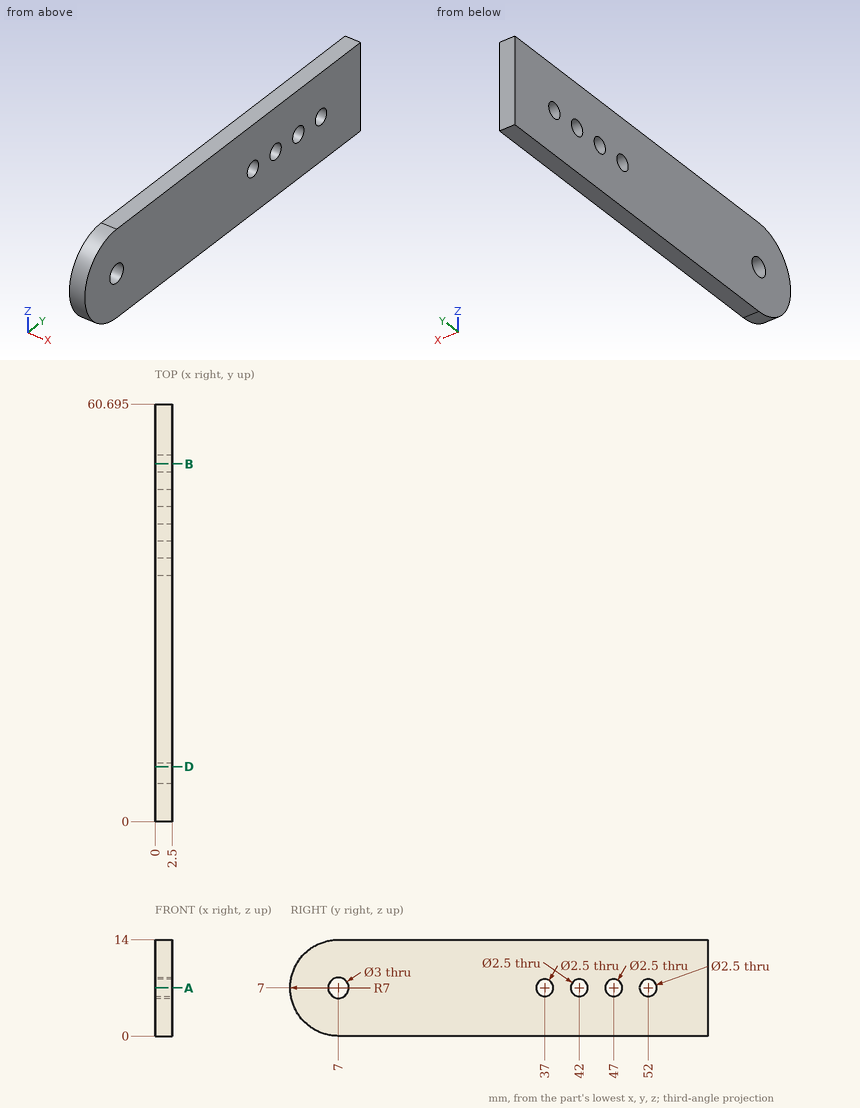
Study the drawing (mm; zero at the part's minimum x, y, z) and answer. Give positions to 0.01 mm unless a question says otherwise; leave off trailing zeros. Loops run counter-clockwise (first coordinate to the right, second up) from the corner with the lowest first, then second, coordinate; pieces in that order, holes last. Notation, with made-up numbers: (46.5, 86) - (70.5, 86) arc R23 ccw to (70.5, 96) - close; hole circle Ø1 at (26.25, 6.5). An arc over 180 degrees is marked (long way). Answer as CSV lines item,"result". Start each with the question number.
1) Straight lines are drawn through the part: L1, parallel to Y at x = 0.2, z = 6.5 (1 decimal); L2, parallel to Z at x = 1.2, y = 42.5 (1 decimal); L3, parallel to Y at x = 2.45, z = 12 (1 decimal). For each, find the intervals that lie inside material, in ascending order. Write a range as from..to.
2) Find section B-B (y = 52). Write down the section's boundary in (x, z).
3) Find section A-A (z = 7). State how many separate pieces and enclosed holes the cut face has, then the cut area to 3 significant figures.
4) Find section D-D (y = 8). Write down the section's boundary in (x, z), then the cut area to 3 significant figures.
Findings below:
1,L1,"0..5.6, 8.4..35.9, 38.1..40.9, 43.1..45.9, 48.1..50.9, 53.1..60.7"
1,L2,"0..5.9, 8.1..14"
1,L3,"2.1..60.7"
2,outline,"(0, 0) - (2.5, 0) - (2.5, 5.75) - (0, 5.75) - close; (0, 8.25) - (2.5, 8.25) - (2.5, 14) - (0, 14) - close"
3,separate pieces,"6"
3,enclosed holes,"0"
3,area,"119 mm^2"
4,outline,"(0, 0) - (2.5, 0) - (2.5, 5.88) - (0, 5.88) - close; (0, 8.12) - (2.5, 8.12) - (2.5, 14) - (0, 14) - close"
4,area,"29.4 mm^2"
